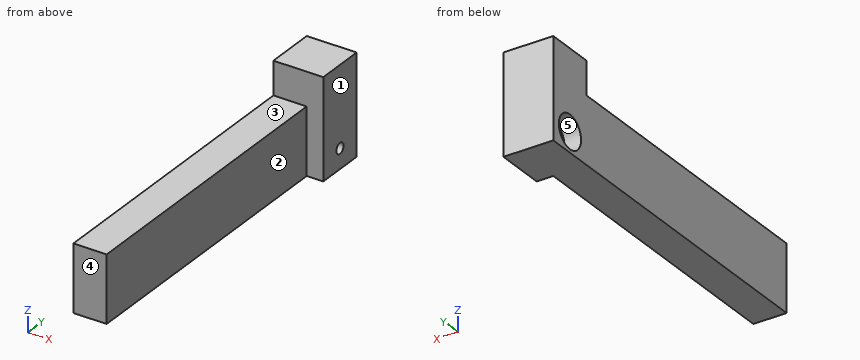
Autodesk Inventor part; units mm, degrees
ref_plane "YZ Plane" through (0, 0, 0) normal (1, 0, 0) x (0, 1, 0)
ref_plane "XZ Plane" through (0, 0, 0) normal (0, 1, 0) x (-1, 0, 0)
ref_plane "XY Plane" through (0, 0, 0) normal (0, 0, 1) x (1, 0, 0)
sketch "base" plane through (0, 0, 0) normal (0, 1, 0) x (-1, 0, 0)
  line L0 (0, 0) -> (0, -20)
  line L1 (0, -20) -> (10, -20)
  line L2 (10, -20) -> (10, 0)
  line L3 (10, 0) -> (0, 0)
  dimension "d186" = 20
  dimension "d187" = 10
extrude "Extrusión29" add sketch "base" along normal blind 90
sketch "Boceto41" plane through (0, 90, 0) normal (0, 1, 0) x (1, 0, 0)
  line L0 (0, 20) -> (5, 20)
  line L1 (5, 20) -> (5, 0)
  line L2 (-10, 0) -> (0, 0)
  line L3 (5, 0) -> (-10, 0)
  line L4 (-10, 0) -> (-10, 20)
  line L5 (-10, 20) -> (5, 20)
  dimension "d190" = 5
extrude "Extrusión30" add sketch "Boceto41" along normal blind 15
sketch "Boceto42" plane through (-10, 0, 0) normal (0, 0, 1) x (1, 0, 0)
  line L0 (15, 90) -> (10, 90)
  line L1 (15, 90) -> (0, 90)
  line L2 (0, 0) -> (0, 105)
  line L3 (0, 90) -> (0, 105)
  line L4 (0, 105) -> (15, 105)
  line L5 (0, 105) -> (15, 105)
  line L6 (15, 105) -> (15, 90)
  point P0 (10, 0)
extrude "Extrusión31" add sketch "Boceto42" along normal blind 10
sketch "Boceto45" plane through (5, 90, -20) normal (1, 0, 0) x (0, 0, -1)
  line L0 (0, -90) -> (0, 15)
  line L1 (0, 0) -> (0, 15)
  line L2 (0, 7.5) -> (-6, 7.5)
  point P0 (-20, -90)
  dimension "d200" = 6
hole "Agujero1" at (5, 97.5, -14) direction (-1, 0, 0) diameter 3.2 end through all
sketch "Boceto51" plane through (-10, 0, -20) normal (-1, 0, 0) x (0, 0, 1)
  circle A0 centre (6, 97.5) radius 1.6
  circle A1 centre (6, 97.5) radius 1.6
  point P0 (20, 0)
hole "Agujero2" at (-10, 97.5, -14) direction (1, 0, 0) diameter 3.2 depth 30 counterbore diameter 10 counterbore depth 5
properties part number "detector curvament fil"
Could you check a few things on this model? Use its own coordinates, in mm. Face numbers are marked on the shaded views. A direction names the side the tool comes from. Coordinates: 2 decimals unless noted, no trailing zeros. Order: outer loops, then holes, each group sorted by start corner. A loop starts at its lowest first (then second) coordinate and runs counter-clockwise, first axis right, second up. Notation, with made-up numbers: M 83.5,-2.75 L 128.5,-2.75 A20 cw 128.5,25.25 Z; hole C 9,48 d3. An arc over 180 degrees is marked long. Use one line per item in the form item = value. Start each with the question number.
1. Suppose I cut it at D-D on z = -7.25. Write out the boundary of the cut face in (x, y).
2. Suppose I cut it at C-C on z = -14. Write out the boundary of the cut face in (x, y), then the cut area to 3 significant figures.
3. Suppose I cut it at B-B on y = 97.5. Write out the boundary of the cut face in (x, z), then the cut area to 3 significant figures.
4. For pin 1 (5 mm diameter, centred on y = 78.5, z = -9.5, fed in from +X); pin 2 (5 mm diameter, centred on x = -6.5, y = 51.5, fed in from +Z); pin 3 (8 mm diameter, centred on y = 97.5, z = -14, fed in from -X), each with a flat end and sliding along its axis, tell me the tip position at first contact or that it passes through.
5. Please list where these lines run through material, in increasing order: line 1 (Z direction, x = 2.25, y = 97.5); line 2 (Y direction, x = 1, z = -14); line 3 (Z direction, x = -7.45, y = 97.5).
6. We'd pull the mould along Z, two halves only. Please class the marked faces 3, 4 and 5: +Z half, -Z half, draft (parallel to the pull), parting line (faces both ways), or undercut.
7. On a 3-axis mill with a long thin cutter (end or side, diameter ignored), from which of +Z, -Z, +X, -X, +Y, -Y can I reach the whole of each face in a straight line? I mean the marked faces 1 and 2. Say none if no direction works.
8. Suppose I cut it at A-A on x = -2.75. Write out the boundary of the cut face in (y, z).
Geometry says:
q1.outline = M -10,0 L 0,0 L 0,90 L 5,90 L 5,105 L -10,105 Z
q2.outline = M -10,0 L 0,0 L 0,90 L 5,90 L 5,95.9 L -5,95.9 L -5,92.5 L -10,92.5 Z; M -10,102.5 L -5,102.5 L -5,99.1 L 5,99.1 L 5,105 L -10,105 Z
q2.area = 1,040 mm^2
q3.outline = M -10,-20 L 5,-20 L 5,-15.6 L -5,-15.6 L -5,-19 L -10,-19 Z; M -10,-9 L -5,-9 L -5,-12.4 L 5,-12.4 L 5,10 L -10,10 Z
q3.area = 368 mm^2
q4.pin_1 = 0
q4.pin_2 = 0
q4.pin_3 = -5
q5.line_1 = -20 to -15.6, -12.4 to 10
q5.line_2 = 90 to 95.9, 99.1 to 105
q5.line_3 = -20 to -19, -9 to 10
q6.face_3 = +Z half
q6.face_4 = draft
q6.face_5 = undercut
q7.face_1 = +Z, -Z, +X, +Y, -Y
q7.face_2 = +Z, -Z, +X, -Y
q8.outline = M 0,-20 L 105,-20 L 105,10 L 90,10 L 90,0 L 0,0 Z; hole C 97.5,-14 d3.2
